```python
from build123d import *

# Parameters (mm, degrees)
BOSS_EXTRUDE1_DEPTH                             = 12
BOSS_EXTRUDE2_START                             = -35
SKETCH1_4_R                                     = 1.1
BOSS_EXTRUDE2_DEPTH                             = 35
SKETCH4_W                                       = 7.2
SKETCH4_H                                       = 7.2
CUT_EXTRUDE1_DEPTH                              = 10
CIRPATTERN1_COUNT                               = 3
FILLET1_R                                       = 3
CSK_FOR_M3_OVAL_HEAD_MACHINE_SCREW1_D           = 3.6
CSK_FOR_M3_OVAL_HEAD_MACHINE_SCREW1_CSINK_D     = 6.3
CSK_FOR_M3_OVAL_HEAD_MACHINE_SCREW1_CSINK_ANGLE = 90


with BuildPart() as part:
    # Sketch1 → Boss-Extrude1 (new body)
    with BuildSketch(Plane.XY):
        with BuildLine():
            ThreePointArc((-5.777817459, -13.842572933), (-3.326773194, -14.626434293), (-0.777817459, -14.979819759))
            Line((-0.777817459, -14.979819759), (-0.777817459, -0.777817459))
            ThreePointArc((-0.777817459, -0.777817459), (-0.420951776, 1.016267486), (1.1, 0))
            ThreePointArc((1.1, 0), (1.016267486, -0.420951776), (0.777817459, -0.777817459))
            Line((0.777817459, -0.777817459), (0.777817459, -14.979819759))
            ThreePointArc((0.777817459, -14.979819759), (3.326773194, -14.626434293), (5.777817459, -13.842572933))
            ThreePointArc((5.777817459, -13.842572933), (12.483334128, -8.316632074), (15, 0))
            ThreePointArc((15, 0), (-8.316632074, 12.483334128), (-5.777817459, -13.842572933))
        make_face()
        with BuildLine():
            Line((-5.777817459, -22.777817459), (-0.777817459, -22.777817459))
            Line((-0.777817459, -22.777817459), (-0.777817459, -14.979819759))
            ThreePointArc((-0.777817459, -14.979819759), (-3.326773194, -14.626434293), (-5.777817459, -13.842572933))
            Line((-5.777817459, -13.842572933), (-5.777817459, -22.777817459))
        make_face()
        with BuildLine():
            ThreePointArc((5.777817459, -13.842572933), (3.326773194, -14.626434293), (0.777817459, -14.979819759))
            Line((0.777817459, -14.979819759), (0.777817459, -22.777817459))
            Line((0.777817459, -22.777817459), (5.777817459, -22.777817459))
            Line((5.777817459, -22.777817459), (5.777817459, -13.842572933))
        make_face()
    extrude(amount=BOSS_EXTRUDE1_DEPTH)

    # Sketch1_4 → Boss-Extrude2 (add)
    with BuildSketch(Plane.XY.offset(BOSS_EXTRUDE2_START)):
        with BuildLine():
            ThreePointArc((-5.777817459, -13.842572933), (-3.326773194, -14.626434293), (-0.777817459, -14.979819759))
            Line((-0.777817459, -14.979819759), (-0.777817459, -0.777817459))
            ThreePointArc((-0.777817459, -0.777817459), (-0.420951776, 1.016267486), (1.1, 0))
            ThreePointArc((1.1, 0), (1.016267486, -0.420951776), (0.777817459, -0.777817459))
            Line((0.777817459, -0.777817459), (0.777817459, -14.979819759))
            ThreePointArc((0.777817459, -14.979819759), (3.326773194, -14.626434293), (5.777817459, -13.842572933))
            ThreePointArc((5.777817459, -13.842572933), (12.483334128, -8.316632074), (15, 0))
            ThreePointArc((15, 0), (-8.316632074, 12.483334128), (-5.777817459, -13.842572933))
        make_face()
        with BuildLine():
            Line((-0.777817459, -0.777817459), (-0.777817459, -14.979819759))
            ThreePointArc((-0.777817459, -14.979819759), (0, -15), (0.777817459, -14.979819759))
            Line((0.777817459, -14.979819759), (0.777817459, -0.777817459))
            ThreePointArc((0.777817459, -0.777817459), (0, -1.1), (-0.777817459, -0.777817459))
        make_face()
        with BuildLine():
            ThreePointArc((-5.777817459, -13.842572933), (-3.326773194, -14.626434293), (-0.777817459, -14.979819759))
            Line((-0.777817459, -14.979819759), (-0.777817459, -0.777817459))
            ThreePointArc((-0.777817459, -0.777817459), (-0.420951776, 1.016267486), (1.1, 0))
            ThreePointArc((1.1, 0), (1.016267486, -0.420951776), (0.777817459, -0.777817459))
            Line((0.777817459, -0.777817459), (0.777817459, -14.979819759))
            ThreePointArc((0.777817459, -14.979819759), (3.326773194, -14.626434293), (5.777817459, -13.842572933))
            ThreePointArc((5.777817459, -13.842572933), (12.483334128, -8.316632074), (15, 0))
            ThreePointArc((15, 0), (-8.316632074, 12.483334128), (-5.777817459, -13.842572933))
        make_face()
        with BuildLine():
            Line((-0.777817459, -0.777817459), (-0.777817459, -14.979819759))
            ThreePointArc((-0.777817459, -14.979819759), (0, -15), (0.777817459, -14.979819759))
            Line((0.777817459, -14.979819759), (0.777817459, -0.777817459))
            ThreePointArc((0.777817459, -0.777817459), (0, -1.1), (-0.777817459, -0.777817459))
        make_face()
        Circle(SKETCH1_4_R)
    extrude(amount=BOSS_EXTRUDE2_DEPTH)

    # Sketch4 → Cut-Extrude1 (cut, symmetric)
    with BuildSketch(Plane(origin=(0, -14.979819759, 0), x_dir=(-1, 0, 0), z_dir=(0, -1, 0))):
        with Locations((2.177817459, 23.6)):
            Rectangle(SKETCH4_W, SKETCH4_H)
    cut_extrude1 = extrude(amount=CUT_EXTRUDE1_DEPTH, both=True, mode=Mode.SUBTRACT)

    # CirPattern1: Cut-Extrude1 ×3 about axis
    cirpattern1_axis = Axis((0, 0, 0), (0, 0, 1))
    for i in range(1, CIRPATTERN1_COUNT):
        add(cut_extrude1.rotate(cirpattern1_axis, i * 360 / CIRPATTERN1_COUNT), mode=Mode.SUBTRACT)

    # Fillet1
    fillet1_edges = [part.edges().sort_by_distance(p)[0] for p in [
        (5.777817459, 13.842572933, -35),
    ]]
    fillet(fillet1_edges, radius=FILLET1_R)

    # CSK for M3 Oval Head Machine Screw1 (through all)
    with Locations(Plane.ZY.offset(5.777817459)):
        with Locations((6.016146397, -18.321749647)):
            CounterSinkHole(CSK_FOR_M3_OVAL_HEAD_MACHINE_SCREW1_D / 2, CSK_FOR_M3_OVAL_HEAD_MACHINE_SCREW1_CSINK_D / 2, counter_sink_angle=CSK_FOR_M3_OVAL_HEAD_MACHINE_SCREW1_CSINK_ANGLE)


solid = part.part
```
Here's how the part is built. I have some questions about the finished solid (model axes, mm). A direction names the side the tool comes from. Coordinates: 2 decimals unless noted, no trailing zeros. Loops run counter-clockwise (first coordinate to the right, second up) from the corner with the lowest first, then second, coordinate; pieces in that order, holes last. Notation, with made-up numbers: (56.25, -37.5) - (108.25, -37.5) arc R26 cw to (108.25, -2.5) - close; hole circle Ø1 at (-28.75, 31). An arc over 180 degrees is marked (long way). Return JSON: item names as keys, results as strings. Group by question number.
Item 1: If we section it at B-B on x = -3: State how many separate pieces and enclosed holes the cut face has, and give its area (3 significant figures).
Item 2: I need wall thicknesses on line 1 (X direction, y = -15, z = 9.5); line 2 (Z direction, x = 8, y = 2); line 3 (X direction, y = 0.5, z = -14.5). Which ranges of each line are inside material? Lowest first, please. Write a range as from..to.
Item 3: Will these pins go through, and if not, where does the flat tip stop? P1, Ø3, axis at x = -9.5, z = -21, coming from the -Y side; P2, Ø1.1, axis at x = -0.5, y = -7.5, coming from the +Z side; P3, Ø13, axis at y = -8, z = 7, coming from the +X side; P4, Ø9.5, axis at y = -14, z = 4.5, coming from the -X side.
Item 4: If we section it at A-A on z = -17: Write out the boundary of the cut face in (x, y).
Item 5: We'd pull the mould along Y, two halves only. Please class faces 5 (the face through (11.09, -0.27, -23.55)), 6 (the face through (3, -22.778, 6)), 7 (the face through (3, -18, 0)): +Y half, -Y half, draft (parallel to the pull), parting line (faces both ways), or undercut.
Item 6: On a 3-axis mill with a long thin cutter (end or side, diameter ignored), from which of +Z, -Z, +X, -X, +Y, -Y can I reach the whole of each face in a straight line? I mean faces 1 (the face through (-5.778, -15, 5)), 2 (the face through (10, 3, -27.2)), 3 (the face through (-0.778, -12, 6)), 4 (the face through (-2, -10, -27.2)). Say none if no direction works.
Calculated:
{
 "1": {"separate pieces": "1", "enclosed holes": "2", "area": "1,370 mm^2"},
 "2": {"line 1": "x = -5.78..-0.78, 0.78..5.78", "line 2": "z = -35..-27.2, -20..12", "line 3": "x = -14.99..14.99"},
 "3": {"P1": "stops at y = -12.69", "P2": "stops at z = 12", "P3": "stops at x = 14.92", "P4": "stops at x = -11.81"},
 "4": {"outline": "circle Ø30 at (0, 0)"},
 "5": {"face 5": "undercut", "face 6": "-Y half", "face 7": "draft"},
 "6": {"face 1": "+Z, -Z, -X, -Y", "face 2": "none", "face 3": "+Z, -Y", "face 4": "-Y"}
}
